The model under review builds one solid part; all positions refer to its coordinate system, in mm. A direction names the side the tool comes from. Give positions to 0.01 mm unless a question says otherwise; leave off trailing zeros. Loops run counter-clockwise (first coordinate to the right, second up) from the corner with the lowest first, then second, coordinate; pieces in that order, holes last. Notation, with made-up numbers: M -10,34 L 49,34 A33 ccw 49,63 Z; hole C 21,58.5 d11. An arc over 180 degrees is marked long. Return JSON: item names as keys, results as strings. Group by question number.
```python
from build123d import *

# Parameters (mm, degrees)
SKETCH1_R           = 2
BOSS_EXTRUDE3_DEPTH = 10
CHAMFER2_SIZE       = 0.5
CUT_EXTRUDE2_DEPTH  = 2


with BuildPart() as part:
    # Sketch1 → Boss-Extrude3 (new body)
    with BuildSketch(Plane(origin=(0, 0, 0), x_dir=(1, 0, 0), z_dir=(0, 1, 0))):
        Circle(SKETCH1_R)
    extrude(amount=-BOSS_EXTRUDE3_DEPTH)

    # Sketch3 → Revolve2 (revolve)
    with BuildSketch(Plane.XY):
        with BuildLine():
            Line((-3.5, 0), (-3.5, 0.3))
            ThreePointArc((-3.5, 0.3), (-1.988393808, 1.6859585), (0, 2.188078318))
            Line((0, 2.188078318), (0, 0))
            Line((0, 0), (-3.5, 0))
        make_face()
    revolve(axis=Axis((0, -2, 0), (0, 1, 0)))

    # Chamfer2
    chamfer2_edges = [part.edges().sort_by_distance(p)[0] for p in [
        (-2, -10, 0),
    ]]
    chamfer(chamfer2_edges, length=CHAMFER2_SIZE)

    # Sketch4 → Cut-Extrude2 (cut)
    with BuildSketch(Plane(origin=(0, 2.188078318, 0), x_dir=(1, 0, 0), z_dir=(0, 1, 0))):
        Polygon((0, 1.732050808), (-1.5, 0.866025404), (-1.5, -0.866025404), (0, -1.732050808), (1.5, -0.866025404), (1.5, 0.866025404), align=None)
    extrude(amount=-CUT_EXTRUDE2_DEPTH, mode=Mode.SUBTRACT)


solid = part.part
```
(1) For pin 1 (1.5 mm diameter, centred on y = -5, z = -1, fed in from +X); pin 2 (3 mm diameter, centred on y = -4.5, z = 2, fed in from -X); pin 3 (1.4 mm diameter, centred on y = 1.5, z = 0, fed in from -X), all flat-tipped, find the tip position at first contact; note any pin that passes through.
(2) Add section B-B (z = 0). Write out the cut boundary in (x, y).
(3) Mouldability with a two-part tool opening along X and no side actions: class faces 3 (the flat face through (0.76, 1.061, -1.293)), 4 (the cylindrical face through (0, -5, 2)), 5 (the flat face through (0, 0.188, 0)), 6 (the flat face through (2, 0, -2)) as released by +X, released by -X, zero draft, split by the parting line, or undercut.
(4) Add section C-C (y = -1). Write out the cut boundary in (x, z), and give its area (3 significant figures).
(5) For faces 1 (the flat face through (0.74, 1.061, 1.305)), 2 (the flat face through (0, -10, 0)), list the 3-axis set-ups (+Z, -Z, +X, -X, +Y, -Y) from which the entire face can be reached by the end or side of a thin tool; tool diameter is ignored.
(6) Add section A-A (y = 1.25). Write out the cut boundary in (x, z).
(7) For probe 1 along X at (y, z) = (-2, 1); probe 2 along Z at (x, y) = (0, -5); probe 3 along Y at (x, z) = (1.25, 0.5), list the stretches that pass through material, from the lowest coordinate up.
(8) Add section D-D (x = -2.5). Write out the cut boundary in (y, z).
Verdict:
{
 "1": {"pin 1": "stops at x = 1.98", "pin 2": "stops at x = -1.94", "pin 3": "stops at x = -3.11"},
 "2": {"outline": "M -3.5,0 L -2,0 L -2,-9.5 L -1.5,-10 L 1.5,-10 L 2,-9.5 L 2,0 L 3.5,0 L 3.5,0.3 A4.19 ccw 1.5,1.91 L 1.5,0.19 L -1.5,0.19 L -1.5,1.91 A4.19 ccw -3.5,0.3 Z"},
 "3": {"face 3": "undercut", "face 4": "split by the parting line", "face 5": "undercut", "face 6": "zero draft"},
 "4": {"outline": "C 0,0 d4", "area": "12.6 mm²"},
 "5": {"face 1": "+Y", "face 2": "+Z, -Z, +X, -X, -Y"},
 "6": {"outline": "C 0,0 d5.28; hole M -1.5,-0.87 L 0,-1.73 L 1.5,-0.87 L 1.5,0.87 L 0,1.73 L -1.5,0.87 Z"},
 "7": {"probe 1": "x = -1.73 to 1.73", "probe 2": "z = -2 to 2", "probe 3": "y = -10 to 0.19"},
 "8": {"outline": "M 0,-2.45 L 0.3,-2.45 A3.36 ccw 0.3,2.45 L 0,2.45 Z"}
}
